The figure shows three views and two pictorial views of one solid part (mm, origin at its lowest corner). Answer the questions. A direction names the side the tool comes from. Round coordinates to 2 decimals unless told otherwise and drop trailing zeros. Order: outer loops, then holes, each group sorted by start corner. A loop starts at its lowest first (then second) coordinate and runs counter-clockwise, first axis right, second up. Notation, with made-up numbers: (59.25, 64.25) -> (83.25, 64.25) arc R26 cw to (83.25, 90.25) -> close; hole circle Ø6 at (41, -20). An arc over 180 degrees is marked (long way). Answer in a Markdown table with one row per item. Add a question column.
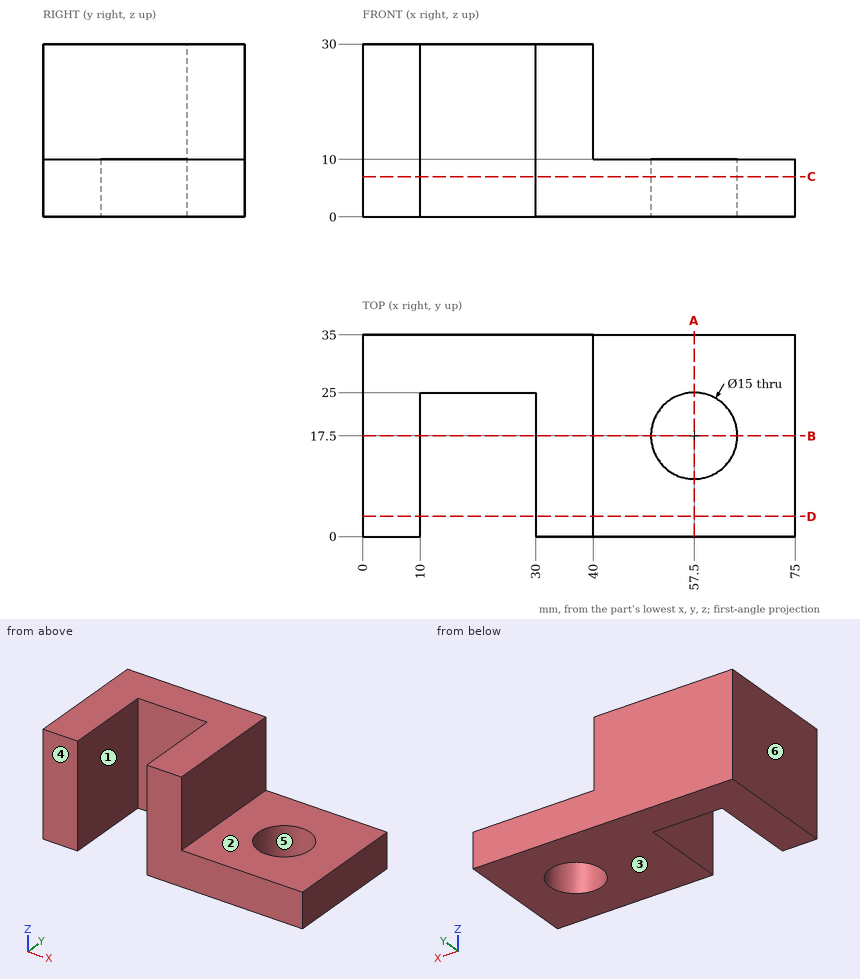
1. The part is cut by section D-D (y = 3.5). Give the vertices of the cut face in (x, z), then the cut area to 3 significant figures.
2. The part is cut by section B-B (y = 17.5). Give the vertices of the cut face in (x, z), then the cut area to 3 significant figures.
3. Straight lines are drawn through the part: line 1 along Y through (x, z) = (57.5, 7.5); line 2 along X through (y, z) = (18, 12); line 3 along X through (y, z) = (13, 2.25). For each, find the intervals that lie inside material, in ascending order.
4. For the marked faces 1, 2 and 3, determine the directions among +Z, -Z, +X, -X, +Y, -Y from which every point of the face is accessible in a straight line to the end or side of a thin tool.
5. The part is cut by section A-A (x = 57.5). Give the vertices of the cut face in (y, z).
6. Each of these flat-tipped pins is pushed along its axis until it touches: pin 1 (16 mm diameter, centred on y = 9, z = 23, fed in from +X); pin 2 (1 mm diameter, centred on x = 19.5, z = 20.5, fed in from -Y); pin 3 (9 mm diameter, centred on x = 57.5, y = 17.5, fed in from -Z). Where does it stop, or does it pass through?
7. The mould has two halves that part along X. Classify the marked faces 4, 5 and 6: released by +X, released by -X, zero draft, split by the parting line, or undercut.
8. The part is cut by section C-C (z = 7). Give the vertices of the cut face in (x, y).
Report:
| question | item | result |
|---|---|---|
| 1 | outline | (0, 0) -> (10, 0) -> (10, 30) -> (0, 30) -> close; (30, 0) -> (75, 0) -> (75, 10) -> (40, 10) -> (40, 30) -> (30, 30) -> close |
| 1 | area | 950 mm^2 |
| 2 | outline | (0, 0) -> (10, 0) -> (10, 30) -> (0, 30) -> close; (30, 0) -> (50, 0) -> (50, 10) -> (40, 10) -> (40, 30) -> (30, 30) -> close; (65, 0) -> (75, 0) -> (75, 10) -> (65, 10) -> close |
| 2 | area | 800 mm^2 |
| 3 | line 1 | y = 0 to 10, 25 to 35 |
| 3 | line 2 | x = 0 to 10, 30 to 40 |
| 3 | line 3 | x = 0 to 10, 30 to 51.5, 63.5 to 75 |
| 4 | face 1 | +Z, -Z, -Y |
| 4 | face 2 | +Z, +X, +Y, -Y |
| 4 | face 3 | -Z, +X, -X, +Y, -Y |
| 5 | outline | (0, 0) -> (10, 0) -> (10, 10) -> (0, 10) -> close; (25, 0) -> (35, 0) -> (35, 10) -> (25, 10) -> close |
| 6 | pin 1 | stops at x = 40 |
| 6 | pin 2 | stops at y = 25 |
| 6 | pin 3 | passes through |
| 7 | face 4 | zero draft |
| 7 | face 5 | undercut |
| 7 | face 6 | released by -X |
| 8 | outline | (0, 0) -> (10, 0) -> (10, 25) -> (30, 25) -> (30, 0) -> (75, 0) -> (75, 35) -> (0, 35) -> close; hole circle Ø15 at (57.5, 17.5) |
